from build123d import *

# Parameters (mm, degrees)
SKETCH1_W             = 44
SKETCH1_H             = 44
SKETCH1_R             = 0.5
SKETCH1_R_2           = 3.5
SKETCH1_H_2           = 5
BOSS_EXTRUDE1_DEPTH   = 3.175
SKETCH3_W             = 6
SKETCH3_H             = 54
SKETCH3_R             = 1.4732
BOSS_EXTRUDE2_DEPTH   = 3.175
M3X0_5_TAPPED_HOLE1_D = 2.5
FILLET1_R             = 1.5875


with BuildPart() as part:
    # Sketch1 → Boss-Extrude1 (new body)
    # profile 1 of 3: a face of its own
    with BuildSketch(Plane(origin=(0, 0, 0), x_dir=(1, 0, 0), z_dir=(0, 1, 0))):
        with Locations((22, -22)):
            Rectangle(SKETCH1_W, SKETCH1_H)
        with Locations(Location((40.93, -16, 0), (0, 0, 270))):
            Circle(SKETCH1_R, mode=Mode.SUBTRACT)
        with Locations(Location((20.93, -16, 0), (0, 0, 270))):
            Circle(SKETCH1_R, mode=Mode.SUBTRACT)
        with Locations(Location((7, -37, 0), (0, 0, 270))):
            Circle(SKETCH1_R_2, mode=Mode.SUBTRACT)
        with Locations(Location((37, -37, 0), (0, 0, 270))):
            Circle(SKETCH1_R_2, mode=Mode.SUBTRACT)
        with Locations(Location((37, -7, 0), (0, 0, 270))):
            Circle(SKETCH1_R_2, mode=Mode.SUBTRACT)
        with Locations(Location((7, -7, 0), (0, 0, 270))):
            Circle(SKETCH1_R_2, mode=Mode.SUBTRACT)
    # profile 2 of 3: a face of its own
    with BuildSketch(Plane(origin=(0, 0, 0), x_dir=(1, 0, 0), z_dir=(0, 1, 0))):
        with Locations((22, 2.5)):
            Rectangle(SKETCH1_W, SKETCH1_H_2)
    # profile 3 of 3: a face of its own
    with BuildSketch(Plane(origin=(0, 0, 0), x_dir=(1, 0, 0), z_dir=(0, 1, 0))):
        with Locations((22, -46.5)):
            Rectangle(SKETCH1_W, SKETCH1_H_2)
    extrude(amount=BOSS_EXTRUDE1_DEPTH)

    # Sketch3 → Boss-Extrude2 (add)
    # profile 1 of 2: a face of its own
    with BuildSketch(Plane(origin=(0, 3.175, 0), x_dir=(1, 0, 0), z_dir=(0, 1, 0))):
        with Locations((-3, -22)):
            Rectangle(SKETCH3_W, SKETCH3_H)
        with Locations(Location((-3, 2, 0), (0, 0, 270))):
            Circle(SKETCH3_R, mode=Mode.SUBTRACT)
        with Locations(Location((-3, -46, 0), (0, 0, 270))):
            Circle(SKETCH3_R, mode=Mode.SUBTRACT)
    # profile 2 of 2: a face of its own
    with BuildSketch(Plane(origin=(0, 3.175, 0), x_dir=(1, 0, 0), z_dir=(0, 1, 0))):
        with Locations((47, -22)):
            Rectangle(SKETCH3_W, SKETCH3_H)
        with Locations(Location((47, -46, 0), (0, 0, 270))):
            Circle(SKETCH3_R, mode=Mode.SUBTRACT)
        with Locations(Location((47, 2, 0), (0, 0, 270))):
            Circle(SKETCH3_R, mode=Mode.SUBTRACT)
    extrude(amount=-BOSS_EXTRUDE2_DEPTH)

    # M3x0.5 Tapped Hole1 (through all)
    with Locations(Plane(origin=(40.93, 3.175, 16), x_dir=(0, 0, 1), z_dir=(0, 1, 0))):
        with Locations((0, 0), (0, -20)):
            Hole(M3X0_5_TAPPED_HOLE1_D / 2)

    # Fillet1
    fillet1_edges = [part.edges().sort_by_distance(p)[0] for p in [
        (-6, 1.5875, -5),
        (-6, 1.5875, 49),
        (50, 1.5875, 49),
        (50, 1.5875, -5),
    ]]
    fillet(fillet1_edges, radius=FILLET1_R)


solid = part.part
Source: CAD feature listing. Evaluate the final solid. Frame: model axes, mm. Give positions to 0.01 mm unless a question says otherwise; leave off trailing zeros. Write each loop counter-clockwise with the first axis right and the second up, starting at its lowest first coordinate (ties: lowest second). Pieces come first, ordered by that corner, then holes. Notation, with made-up numbers: M -3,-1.5 L 14,-1.5 A25 ccw 14,31.5 Z; hole C 72.5,43 d2. An arc over 180 degrees is marked long. Return JSON: item names as keys, results as strings. Group by question number.
1) Cut plane A-A, the plane x = -3. Output: boundary loops of the cut face in (y, z) (3 decimals).
2) Draft query along X for faces 1 (the face through (39.71, 1.57, 16.27)), 2 (the face through (22, 3.175, 22)), 3 (the face through (-5.55, 1.57, -4.52)). Return one class per face: released by +X, released by -X, zero draft, split by the parting line, or undercut.
3) Cut plane B-B, the plane z = 7. Output: boundary loops of the cut face in (x, y) (3 decimals), then the cut area to 3 significant figures.
4) Ray query, L1, parallel to X at y = 0.9, z = 7; L2, parallel to X at y = 0.3, z = -2; L3, parallel to Z at x = 40, y = 1.3. Return the intervals inside material, ascending.
5) Cut plane C-C, the plane y = 0.55. Give the number of separate pieces and of enclosed holes in the cut face, then the cut area to 3 significant figures.
6) First-contact query: pin 1 Ø3.5 at (x, z) = (-3, 46) entering from -Y; pin 2 Ø2.5 at (x, z) = (47, -2) entering from +Y (3 decimals). Flat tips, straight axial feed; report the tip coordinate or a pass-through.
Data:
{
 "1": {"outline": "M 0,-5 L 3.175,-5 L 3.175,-3.473 L 0,-3.473 Z; M 0,-0.527 L 3.175,-0.527 L 3.175,44.527 L 0,44.527 Z; M 0,47.473 L 3.175,47.473 L 3.175,49 L 0,49 Z"},
 "2": {"face 1": "undercut", "face 2": "zero draft", "face 3": "released by -X"},
 "3": {"outline": "M -6,0 L 3.5,0 L 3.5,3.175 L -6,3.175 Z; M 10.5,0 L 33.5,0 L 33.5,3.175 L 10.5,3.175 Z; M 40.5,0 L 50,0 L 50,3.175 L 40.5,3.175 Z", "area": "133 mm²"},
 "4": {"L1": "x = -6 to 3.5, 10.5 to 33.5, 40.5 to 50", "L2": "x = -6 to -4.47, -1.53 to 45.53, 48.47 to 50", "L3": "z = -5 to 5.2, 8.8 to 15.16, 16.84 to 35.2, 38.8 to 49"},
 "5": {"separate pieces": "1", "enclosed holes": "10", "area": "2,830 mm²"},
 "6": {"pin 1": "stops at y = 0", "pin 2": "passes through"}
}
